```python
from build123d import *

# Parameters (mm, degrees)
F0_R     = 19.05
F1_DEPTH = 38.1
F0_R_2   = 6.35
F2_DEPTH = 31.75
F3_DEPTH = 25.4


with BuildPart() as f1:
    # F0 (on Top) → F1 (new body)
    with BuildSketch(Plane.XY):
        with BuildLine():
            ThreePointArc((2.552861, -25.271385), (18.841479, -17.034044), (25.4, 0))
            ThreePointArc((25.4, 0), (18.841479, 17.034044), (2.552861, 25.271385))
            ThreePointArc((2.552861, 25.271385), (-25.4, 0), (2.552861, -25.271385))
        make_face()
        Circle(F0_R, mode=Mode.SUBTRACT)
    extrude(amount=F1_DEPTH)



with BuildPart() as f2:
    # F0 (on Top) → F2 (new body)
    with BuildSketch(Plane.XY):
        with BuildLine():
            ThreePointArc((139.7, 0), (135.980256, 8.980256), (127, 12.7))
            ThreePointArc((127, 12.7), (114.3, 0), (127, -12.7))
            ThreePointArc((127, -12.7), (135.980256, -8.980256), (139.7, 0))
        make_face()
        with Locations((127, 0)):
            Circle(F0_R_2, mode=Mode.SUBTRACT)
    extrude(amount=F2_DEPTH)


with BuildPart() as f1_1:
    add(f1.part)

    add(f2.part)  # F3 merges F2
    # F0 (on Top) → F3 (join)
    with BuildSketch(Plane.XY):
        with BuildLine():
            ThreePointArc((2.552861, 25.271385), (18.841479, 17.034044), (25.4, 0))
            ThreePointArc((25.4, 0), (18.841479, -17.034044), (2.552861, -25.271385))
            Line((2.552861, -25.271385), (127, -12.7))
            ThreePointArc((127, -12.7), (114.3, 0), (127, 12.7))
            Line((127, 12.7), (2.552861, 25.271385))
        make_face()
        with BuildLine():
            ThreePointArc((88.9, 6.35), (95.25, 0), (88.9, -6.35))
            Line((88.9, -6.35), (38.1, -6.35))
            ThreePointArc((38.1, -6.35), (31.75, 0), (38.1, 6.35))
            Line((38.1, 6.35), (88.9, 6.35))
        make_face(mode=Mode.SUBTRACT)
    extrude(amount=F3_DEPTH)


solid = f1_1.part
```
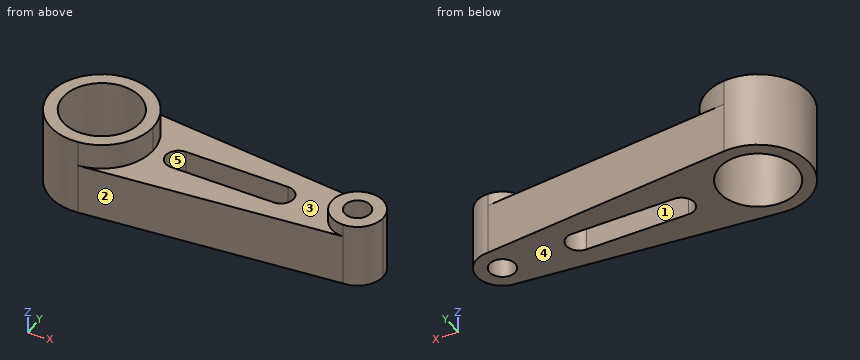
Part model, mm, in its own coordinate system. Face numbers are marked on the shaded views. A direction names the side the tool comes from. Give positions to 0.01 mm unless a question says otherwise; leave off trailing zeros. Write each loop counter-clockwise with the first axis right and the second up, starting at its lowest first coordinate (ties: lowest second). Pieces come first, ordered by that corner, then holes. Notation, with made-up numbers: (-19, -17) -> (-5, -17) arc R18 cw to (-5, -10) -> close; hole circle Ø8 at (22, -15). An arc over 180 degrees is marked (long way). Put each result on its own line as item: value. Start each with the question number.
Item 1: Which spindle directions (+Z, -Z, +X, -X, +Y, -Y) get a long thin tool onto all of the face, cutting with end or side? Do the marked faces 4 and 5. Say none if no direction does.
Item 2: Cut at B-B (z = 10). List the corners of the cut face in (x, y), then the cut area to 3 significant figures.
Item 3: Wall check: L1, parallel to Y at x = 0, z = 20; L2, parallel to Y at x = 127, z = 25; L3, parallel to X at y = -3.5, z = 15. Give the ranges that are in metal, low to high. Write a range as [from, to].
Item 4: Cut at C-C (y = -8). List the corners of the cut face in (x, z), then the cut area to 3 significant figures.
Item 5: Cut at D-D (y = -21). List the corners of the cut face in (x, z).
Item 6: Pin check, flat tips, straight feed: pin 1 Ø10 at (x, y) = (127, 0) entering from -Z; pin 2 Ø8 at (x, z) = (123, 17) entering from -Y; pin 3 Ø8 at (y, z) = (-17.5, 13.5) entering from -X; pin 4 Ø3 at (x, z) = (87.5, 9) entering from -Y. Stop position of each tip, or through.
Item 7: Pull direction Y, two halves, no side cores. Call the marked faces 1, 2 and 3: pulls with the +Y half, pulls with the -Y half, needs draft (parallel to the pull), parting line crosses it, or undercut.
Item 8: Cut at A-A (x = 0). List the corners of the cut face in (y, z).
Answer list:
1. face 4: -Z, +X, -X, +Y, -Y
1. face 5: +Z, -Z
2. outline: (2.55, -25.27) -> (127, -12.7) arc R12.7 ccw to (127, 12.7) -> (2.55, 25.27) arc R25.4 ccw (long way) to start; hole circle Ø38.1 at (0, 0); hole (38.1, -6.35) -> (88.9, -6.35) arc R6.35 ccw to (88.9, 6.35) -> (38.1, 6.35) arc R6.35 ccw to start; hole circle Ø12.7 at (127, 0)
2. area: 4,080 mm2
3. L1: y = [-25.4, -19.05], [19.05, 25.4]
3. L2: y = [-12.7, -6.35], [6.35, 12.7]
3. L3: x = [-25.16, -18.73], [18.73, 32.8], [94.2, 121.7], [132.3, 139.21]
4. outline: (-24.11, 0) -> (-17.29, 0) -> (-17.29, 38.1) -> (-24.11, 38.1) -> close; (17.29, 0) -> (136.86, 0) -> (136.86, 31.75) -> (117.14, 31.75) -> (117.14, 25.4) -> (24.11, 25.4) -> (24.11, 38.1) -> (17.29, 38.1) -> close
4. area: 3,510 mm2
5. outline: (-14.29, 0) -> (44.84, 0) -> (44.84, 25.4) -> (14.29, 25.4) -> (14.29, 38.1) -> (-14.29, 38.1) -> close
6. pin 1: passes through
6. pin 2: stops at y = -13.51
6. pin 3: stops at x = -21.52
6. pin 4: stops at y = -16.84
7. face 1: undercut
7. face 2: pulls with the -Y half
7. face 3: needs draft
8. outline: (-25.4, 0) -> (-19.05, 0) -> (-19.05, 38.1) -> (-25.4, 38.1) -> close; (19.05, 0) -> (25.4, 0) -> (25.4, 38.1) -> (19.05, 38.1) -> close
